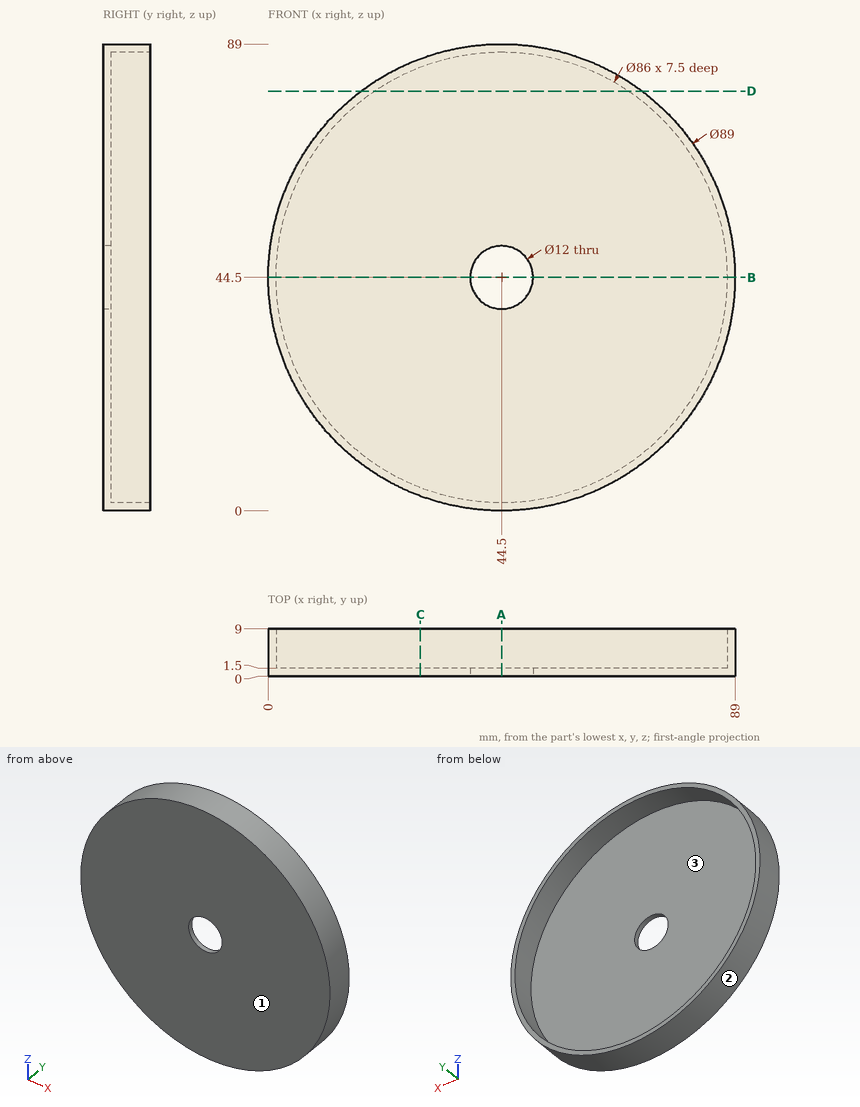
Print and shaded views of the part. All mm, measured from the part's lowest x, y and z. Coordinates: 2 decimals unless noted, no trailing zeros. Order: outer loops, then holes, each group sorted by start corner. A loop starts at its lowest first (then second) coordinate and runs counter-clockwise, first axis right, second up. Notation, with made-up numbers: M 83,52.5 L 135,52.5 A37 cw 135,89.5 Z; hole C 82.5,78 d8. An arc over 180 degrees is marked long. One line per question, with ' | ' between items. Start each with the question number.
Q1. Saw through at B-B (z = 44.5). List the corners of the cut face in (x, y).
Q2. Probe L1, parallel to X at y = 1.1, z = 44.5; L2, parallel to X at y = 6.5, z = 44.5. List the from-to ranges inside material, lowest first. Write a range as from..to.
Q3. Saw through at C-C (x = 29). List the corners of the cut face in (y, z), then the cut area to 3 significant figures.
Q4. Flat gauge pins, fed straight in: pin 1 Ø4 at (x, y) = (29.5, 7.5) entering from +Z; pin 2 Ø19 at (x, z) = (44.5, 44.5) entering from +Y; pin 3 Ø1.5 at (y, z) = (4.5, 68.5) entering from -X. Where does each tip first touch, or does it go through?
Q5. Saw through at D-D (z = 80). List the corners of the cut face in (x, y), then the cut area to 3 significant figures.
Q6. Two-plate mould, pull along Z, no slides. Class the marked faces 1, 2 and 3: +Z half, -Z half, draft (parallel to the pull), parting line (faces both ways), or undercut.
Q7. Saw through at A-A (x = 44.5). List the corners of the cut face in (y, z).
Check values:
1) outline: M 0,0 L 38.5,0 L 38.5,1.5 L 1.5,1.5 L 1.5,9 L 0,9 Z; M 50.5,0 L 89,0 L 89,9 L 87.5,9 L 87.5,1.5 L 50.5,1.5 Z
2) L1: x = 0..38.5, 50.5..89 | L2: x = 0..1.5, 87.5..89
3) outline: M 0,2.79 L 9,2.79 L 9,4.39 L 1.5,4.39 L 1.5,84.61 L 9,84.61 L 9,86.21 L 0,86.21 Z | area: 149 mm2
4) pin 1: stops at z = 87.06 | pin 2: stops at y = 1.5 | pin 3: stops at x = 6.56
5) outline: M 17.67,0 L 71.33,0 L 71.33,9 L 68.76,9 L 68.76,1.5 L 20.24,1.5 L 20.24,9 L 17.67,9 Z | area: 119 mm2
6) face 1: draft | face 2: parting line | face 3: undercut
7) outline: M 0,0 L 9,0 L 9,1.5 L 1.5,1.5 L 1.5,38.5 L 0,38.5 Z; M 0,50.5 L 1.5,50.5 L 1.5,87.5 L 9,87.5 L 9,89 L 0,89 Z
